Work out the finished part from the listing and answer in its coordinate system (mm). A direction names the side the tool comes from. Coordinates: 2 decimals unless noted, no trailing zeros. Loops run counter-clockwise (first coordinate to the right, second up) from the corner with the lowest first, then second, coordinate; pieces in that order, holes last. Notation, with made-up numbers: (34.25, 68) -> (89.25, 68) arc R14 ccw to (89.25, 79) -> close; hole circle Ø10 at (-34, 72.25). An arc over 180 degrees is marked (long way). Use a Markdown table: item, result. Add a question column.
```python
from build123d import *

# Parameters (mm, degrees)
SKETCH1_W           = 57.5
SKETCH1_H           = 3.408146715
SKETCH1_W_2         = 10
SKETCH1_H_2         = 3
SKETCH1_R           = 1.6
BOSS_EXTRUDE1_DEPTH = 3
SKETCH3_W           = 8.1
SKETCH3_H           = 3.2
SKETCH3_W_2         = 10.1
SKETCH3_H_2         = 3.3
SKETCH3_W_3         = 19.7
SKETCH3_W_4         = 19.5
SKETCH3_H_3         = 3
CUT_EXTRUDE1_DEPTH  = 3
SKETCH4_R           = 0.5
CUT_EXTRUDE2_DEPTH  = 3
SKETCH6_R           = 1.6
BOSS_EXTRUDE2_DEPTH = 3
SKETCH6_2_R         = 1.6
CUT_EXTRUDE3_DEPTH  = 3
CUT_EXTRUDE4_DEPTH  = 3
FILLET1_R           = 2
CUT_EXTRUDE5_DEPTH  = 3
EXTRUDE_THIN1_DEPTH = 3
FILLET2_R           = 1
BOSS_EXTRUDE3_DEPTH = 3
FILLET3_R           = 1


with BuildPart() as part:
    # Sketch1 → Boss-Extrude1 (new body)
    # profile 1 of 4: a face of its own
    with BuildSketch(Plane(origin=(0, 0, 0), x_dir=(1, 0, 0), z_dir=(0, 1, 0))):
        with Locations((15.75, 7.704073358)):
            Rectangle(SKETCH1_W, SKETCH1_H)
    # profile 2 of 4: a face of its own
    with BuildSketch(Plane(origin=(0, 0, 0), x_dir=(1, 0, 0), z_dir=(0, 1, 0))):
        with Locations((0, 4.5)):
            Rectangle(SKETCH1_W_2, SKETCH1_H_2)
    # profile 3 of 4: a face of its own
    with BuildSketch(Plane(origin=(0, 0, 0), x_dir=(1, 0, 0), z_dir=(0, 1, 0))):
        with Locations((29.5, 4.5)):
            Rectangle(SKETCH1_W_2, SKETCH1_H_2)
    # profile 4 of 4: a face of its own
    with BuildSketch(Plane(origin=(0, 0, 0), x_dir=(1, 0, 0), z_dir=(0, 1, 0))):
        Polygon((5, 3), (-5, 3), (-13, 3), (-13, -21.846492531), (44.5, -21.846492531), (44.5, 3), (34.5, 3), (24.5, 3), align=None)
        with Locations(Location((0, 0, 0), (0, 0, 270))):
            Circle(SKETCH1_R, mode=Mode.SUBTRACT)
        with Locations(Location((20, 0, 0), (0, 0, 270))):
            Circle(SKETCH1_R, mode=Mode.SUBTRACT)
    extrude(amount=BOSS_EXTRUDE1_DEPTH)

    # Sketch3 → Cut-Extrude1 (cut)
    # profile 1 of 3: a face of its own
    with BuildSketch(Plane(origin=(0, 3, 0), x_dir=(1, 0, 0), z_dir=(0, 1, 0))):
        with Locations((-8.95, 4.5)):
            Rectangle(SKETCH3_W, SKETCH3_H)
    # profile 2 of 3: a face of its own
    with BuildSketch(Plane(origin=(0, 3, 0), x_dir=(1, 0, 0), z_dir=(0, 1, 0))):
        with Locations((39.45, 4.55)):
            Rectangle(SKETCH3_W_2, SKETCH3_H_2)
    # profile 3 of 3: a face of its own
    with BuildSketch(Plane(origin=(0, 3, 0), x_dir=(1, 0, 0), z_dir=(0, 1, 0))):
        with Locations((14.75, 4.5)):
            Rectangle(SKETCH3_W_3, SKETCH3_H)
        with Locations((14.75, 4.5)):
            Rectangle(SKETCH3_W_4, SKETCH3_H_3, mode=Mode.SUBTRACT)
    extrude(amount=-CUT_EXTRUDE1_DEPTH, mode=Mode.SUBTRACT)

    # Sketch4 → Cut-Extrude2 (cut)
    with BuildSketch(Plane(origin=(0, 3, 0), x_dir=(1, 0, 0), z_dir=(0, 1, 0))):
        with Locations((-4.9, 6.1)):
            Circle(SKETCH4_R)
        with Locations((-4.9, 2.9)):
            Circle(SKETCH4_R)
        with Locations((4.9, 6.1)):
            Circle(SKETCH4_R)
        with Locations((4.9, 2.9)):
            Circle(SKETCH4_R)
        with Locations((24.6, 6.1)):
            Circle(SKETCH4_R)
        with Locations((24.6, 2.9)):
            Circle(SKETCH4_R)
        with Locations((34.4, 2.9)):
            Circle(SKETCH4_R)
        with Locations((34.4, 6.2)):
            Circle(SKETCH4_R)
    extrude(amount=-CUT_EXTRUDE2_DEPTH, mode=Mode.SUBTRACT)

    # Sketch6 → Boss-Extrude2 (add)
    with BuildSketch(Plane(origin=(0, 3, 0), x_dir=(1, 0, 0), z_dir=(0, 1, 0))):
        Polygon((-6.176738334, -4.232762247), (37.924895048, -21.846492531), (24.176946138, -45.658638544), (-16.52624784, -22.158638544), align=None)
        with Locations(Location((22.712844523, -40.194536929, 0), (0, 0, 270))):
            Circle(SKETCH6_R, mode=Mode.SUBTRACT)
        with Locations(Location((27.212844523, -32.400308295, 0), (0, 0, 270))):
            Circle(SKETCH6_R, mode=Mode.SUBTRACT)
        with Locations((-11.062146225, -20.694536929)):
            Circle(SKETCH6_R, mode=Mode.SUBTRACT)
        with Locations((-6.562146225, -12.900308295)):
            Circle(SKETCH6_R, mode=Mode.SUBTRACT)
    extrude(amount=-BOSS_EXTRUDE2_DEPTH)

    # Sketch6<2> → Cut-Extrude3 (cut)
    with BuildSketch(Plane(origin=(0, 3, 0), x_dir=(1, 0, 0), z_dir=(0, 1, 0))):
        with Locations(Location((-6.562146225, -12.900308295, 0), (0, 0, 270))):
            Circle(SKETCH6_2_R)
        with BuildLine():
            ThreePointArc((-12.172550786, -21.846492531), (-11.062146225, -22.294536929), (-9.951741663, -21.846492531))
            Line((-9.951741663, -21.846492531), (-12.172550786, -21.846492531))
        make_face()
        with BuildLine():
            Line((-12.172550786, -21.846492531), (-9.951741663, -21.846492531))
            ThreePointArc((-9.951741663, -21.846492531), (-9.589623339, -21.320377444), (-9.462146225, -20.694536929))
            ThreePointArc((-9.462146225, -20.694536929), (-11.68798674, -19.222014043), (-12.172550786, -21.846492531))
        make_face()
    extrude(amount=-CUT_EXTRUDE3_DEPTH, mode=Mode.SUBTRACT)

    # Sketch8 → Cut-Extrude4 (cut)
    with BuildSketch(Plane(origin=(0, 3, 0), x_dir=(1, 0, 0), z_dir=(0, 1, 0))):
        Polygon((37.924895048, -21.846492531), (47.152165502, -5.864391291), (51.952331521, -20.765599638), (44.5, -26.059092388), align=None)
    extrude(amount=-CUT_EXTRUDE4_DEPTH, mode=Mode.SUBTRACT)

    # Fillet1
    fillet1_edges = [part.edges().sort_by_distance(p)[0] for p in [
        (-16.52624784, 1.5, 22.158638544),
        (24.176946138, 1.5, 45.658638544),
        (44.5, 1.5, 10.45807669),
        (-13, 1.5, -9.408146715),
        (44.5, 1.5, -9.408146715),
    ]]
    fillet(fillet1_edges, radius=FILLET1_R)

    # Sketch9 → Cut-Extrude5 (cut)
    with BuildSketch(Plane(origin=(0, 3, 0), x_dir=(1, 0, 0), z_dir=(0, 1, 0))):
        Polygon((1, -5.1), (32.5, -5.1), (32.5, -11.242686381), (19.0166921, -34.596460718), (-4.365993802, -21.096460718), (1, -11.802286819), align=None)
    extrude(amount=-CUT_EXTRUDE5_DEPTH, mode=Mode.SUBTRACT)

    # Sketch10 → Extrude-Thin1 (add)
    with BuildSketch(Plane(origin=(0, 3, 0), x_dir=(1, 0, 0), z_dir=(0, 1, 0))):
        Polygon((-4.02917863, -23.038408895), (33.945296414, -6.53815934), (32.351236334, -2.869512115), (-5.623238711, -19.369761671), align=None)
        Polygon((-1.3111598, -5.755729233), (17.608558315, -36.351129247), (21.010628303, -34.247342235), (2.090910189, -3.651942221), align=None)
    extrude(amount=-EXTRUDE_THIN1_DEPTH)

    # Fillet2
    fillet2_edges = [part.edges().sort_by_distance(p)[0] for p in [
        (1, 1.5, 11.802286819),
        (32.5, 1.5, 11.242686381),
        (15.139105711, 1.5, 32.357735172),
        (-2.302171748, 1.5, 22.288008936),
        (20.083687523, 1.5, 32.748370433),
        (32.5, 1.5, 7.166153578),
        (2.986366531, 1.5, 5.1),
        (27.217883275, 1.5, 5.1),
        (-2.614232793, 1.5, 18.062321647),
        (4.411323294, 1.5, 15.009654597),
        (8.118301247, 1.5, 13.398939472),
        (10.244069028, 1.5, 16.836554938),
        (6.537091075, 1.5, 18.447270063),
    ]]
    fillet(fillet2_edges, radius=FILLET2_R)

    # Sketch11 → Boss-Extrude3 (add)
    with BuildSketch(Plane(origin=(0, 3, 0), x_dir=(1, 0, 0), z_dir=(0, 1, 0))):
        Polygon((0.814899894, -12.122889607), (2.271586452, -9.599834478), (-0.508630479, -8.514382996), align=None)
    extrude(amount=-BOSS_EXTRUDE3_DEPTH)

    # Fillet3
    fillet3_edges = [part.edges().sort_by_distance(p)[0] for p in [
        (1.689467225, 1.5, 10.608094556),
    ]]
    fillet(fillet3_edges, radius=FILLET3_R)


solid = part.part
```
Item 1: For a pull along Z with two mould halves and no side action, classify faces 1 (the face through (13.9, 0, 11.3)), 2 (the face through (43.899, 1.521, -8.838)), 3 (the face through (-15.72, 1.48, 21.97)), 4 (the face through (-7.17, 1.52, 14.38)) as +Z half, -Z half, draft (parallel to the pull), parting line (faces both ways), or undercut.
Item 2: For faces 5 (the face through (44.5, 1, 4)), 6 (the face through (-9, 2, -6.1)), 7 (the face through (10.752, 1.479, 16.983)), 8 (the face through (40, 2, -2.9)), determine the directions among +Z, -Z, +X, -X, +Y, -Y from which every point of the face is accessible in a straight line to the end or side of a thin tool.
Item 3: Section A-A (z = 0) is taken. Determine the outline of the cut face in (x, y), then the cut area to 3 significant figures.
Item 4: Given pin 1 (0.7 mm diameter, centred on y = 2, z = -4.5, fed in from +X); pin 2 (1.8 mm diameter, centred on y = 2, z = 10.5, fed in from -X); pin 3 (1 mm diameter, centred on x = 27, y = 2, fed in from +Z) (3 decimals), each flat-ended and moving along its own axis, determine where each tip first touches the part or whether it passes through.
Item 5: Find the intervals of material crossed by probe 1 along X at (y, z) = (1, 8.5); probe 2 along Z at (x, y) = (2, 2.5); probe 3 along X at (y, z) = (1.05, 19), in increasing order.
Item 6: Section D-D (x = 39) is taken. Determine the outline of the cut face in (y, z).
Item 7: Section B-B (x = 20) is taken. Determine the outline of the cut face in (y, z).
Item 8: Section C-C (z = 39.5) is taken. Determine the outline of the cut face in (x, y), then the cut area to 3 significant figures.
Output:
| question | item | result |
|---|---|---|
| 1 | face 1 | draft |
| 1 | face 2 | -Z half |
| 1 | face 3 | parting line |
| 1 | face 4 | undercut |
| 2 | face 5 | +Z, -Z, +X, +Y, -Y |
| 2 | face 6 | -X, +Y, -Y |
| 2 | face 7 | +Y, -Y |
| 2 | face 8 | +X, +Y, -Y |
| 3 | outline | (-13, 0) -> (-1.6, 0) -> (-1.6, 3) -> (-13, 3) -> close; (1.6, 0) -> (18.4, 0) -> (18.4, 3) -> (1.6, 3) -> close; (21.6, 0) -> (44.5, 0) -> (44.5, 3) -> (21.6, 3) -> close |
| 3 | area | 153 mm2 |
| 4 | pin 1 | stops at x = 34.4 |
| 4 | pin 2 | stops at x = -13 |
| 4 | pin 3 | stops at z = 41.635 |
| 5 | probe 1 | x = -13 to 5.09, 19.39 to 29.43, 32.48 to 44.5 |
| 5 | probe 2 | z = -9.41 to 11.6, 16.06 to 20.42, 24.77 to 32.85 |
| 5 | probe 3 | x = -14.7 to 5.27, 6.85 to 11.58, 28.02 to 39.57 |
| 6 | outline | (0, -9.41) -> (3, -9.41) -> (3, -6.2) -> (0, -6.2) -> close; (0, -2.9) -> (3, -2.9) -> (3, 19.98) -> (0, 19.98) -> close |
| 7 | outline | (0, -9.41) -> (3, -9.41) -> (3, -6.1) -> (0, -6.1) -> close; (0, -2.9) -> (3, -2.9) -> (3, -1.6) -> (0, -1.6) -> close; (0, 1.6) -> (3, 1.6) -> (3, 5.1) -> (0, 5.1) -> close; (0, 8.24) -> (3, 8.24) -> (3, 12.6) -> (0, 12.6) -> close; (0, 31.8) -> (3, 31.8) -> (3, 43.25) -> (0, 43.25) -> close |
| 8 | outline | (13.51, 0) -> (21.27, 0) -> (21.27, 3) -> (13.51, 3) -> close; (24.15, 0) -> (27.73, 0) -> (27.73, 3) -> (24.15, 3) -> close |
| 8 | area | 34.0 mm2 |
